Part model, mm, in its own coordinate system. A direction names the side the tool comes from. Round coordinates to 2 decimals unless told otherwise and drop trailing zeros. Write each loop counter-clockwise with the first axis right and the second up, starting at its lowest first coordinate (ties: lowest second). Pieces come first, ordered by that corner, then holes. Notation, with made-up numbers: M 35,-34.5 L 70,-34.5 A16 ccw 70,-4.5 Z; hole C -36,58.5 d11. An arc over 180 degrees is marked long. Answer as a JSON object with one key per item and string values. Group by question number.
1. Band-saw the part on C-C, the plane x = 15. Write the cut outline in (y, z) (3 decimals), plus the area to 3 significant figures.
2. Drop a flat-ended pin along its axis: pin 1 (6 mm diameter, centred on x = 0, y = 15.875, fed in from -Z). Give the stop position or say it passes through.
3. Which spindle directions (+Z, -Z, +X, -X, +Y, -Y) get a long thin tool onto all of the face, cutting with end or side? Do faces 1 (the face through (49.91, -3.63, 2.18)), 2 (the face through (-6, -17.78, 0)), 3 (the face through (0, -9.525, 4)). Say none if no direction does.
4. Band-saw the part on B-B, the plane x = 26.67. Write the cut outline in (y, z) (3 decimals).
5. Two-plate mould, pull along Z, no slides. Class faces 4 (the face through (43, 1, 3.429)), 5 (the face through (26.015, -15.274, 3.658)), 6 (the face through (6, -17.78, 0)): +Z half, -Z half, draft (parallel to the pull), parting line (faces both ways), or undercut.
6. Drill centre lines: line 1 (Y direction, x = -22.86, z = 3.15) (3 decimals); line 2 (Y direction, x = -17.78, z = 5.25) (3 decimals); line 3 (Y direction, x = 26.67, z = 3.8) (3 decimals). Where is each one in solid material? Low to high. Write a range as from..to.
7. Band-saw the part on A-A, the plane x = 0. Write the cut outline in (y, z) (3 decimals), plus the area to 3 significant figures.
8. Band-saw the part on D-D, the plane y = -2. Write the cut outline in (x, z) (3 decimals).
from build123d import *

# Parameters (mm, degrees)
F1_DEPTH  = 6.35
F2_W      = 50.8
F2_H      = 19.05
F2_R      = 5.08
F2_R_2    = 3.175
F2_R_3    = 0.635
F2_R_4    = 1.905
F2_R_5    = 1.27
F2_R_6    = 0.889
F3_DEPTH  = 12.7
F4_W      = 35.56
F4_H      = 1.778
F5_DEPTH  = 76.2
F6_W      = 10.16
F6_H      = 2.54
F7_DEPTH  = 10.16
F8_R      = 5.07999
F9_R      = 3.175
F10_DEPTH = 25.4


# Not quite as in the source:
# - a fillet or chamfer is up to 0.001 mm smaller than in the source, because OpenCascade refuses the exact size


with BuildPart() as f1:
    # F0 (on Top) → F1 (new body, symmetric)
    with BuildSketch(Plane.XY):
        with BuildLine():
            Line((38.735, 22.225), (-38.735, 22.225))
            ThreePointArc((-38.735, 22.225), (-40.5310512242, 21.4810512242), (-41.275, 19.685))
            Line((-41.275, 19.685), (-41.275, -19.685))
            ThreePointArc((-41.275, -19.685), (-40.5310512242, -21.4810512242), (-38.735, -22.225))
            Line((-38.735, -22.225), (38.735, -22.225))
            ThreePointArc((38.735, -22.225), (40.5310512242, -21.4810512242), (41.275, -19.685))
            Line((41.275, -19.685), (41.275, 19.685))
            ThreePointArc((41.275, 19.685), (40.5310512242, 21.4810512242), (38.735, 22.225))
        make_face()
    extrude(amount=F1_DEPTH, both=True)

    # F2 (on face) → F3 (cut, through all)
    with BuildSketch(Plane.XY.offset(6.35)):
        Rectangle(F2_W, F2_H)
        with Locations((0, 15.875)):
            Circle(F2_R)
        with Locations((-10.16, 15.875)):
            Circle(F2_R_2)
        with Locations((-29.972, 15.875)):
            Circle(F2_R_3)
        with Locations((-17.78, 15.875)):
            Circle(F2_R_4)
        with Locations((-22.86, 15.875)):
            Circle(F2_R_5)
        with Locations((-26.67, 15.875)):
            Circle(F2_R_6)
        with Locations((29.972, 15.875)):
            Circle(F2_R_3)
        with Locations((22.86, 15.875)):
            Circle(F2_R_5)
        with Locations((26.67, 15.875)):
            Circle(F2_R_6)
        with Locations((17.78, 15.875)):
            Circle(F2_R_4)
        with Locations((10.16, 15.875)):
            Circle(F2_R_2)
        with Locations((29.972, -15.875)):
            Circle(F2_R_3)
        with Locations((0, -15.875)):
            Circle(F2_R)
        with Locations((26.67, -15.875)):
            Circle(F2_R_6)
        with Locations((-22.86, -15.875)):
            Circle(F2_R_5)
        with Locations((-29.972, -15.875)):
            Circle(F2_R_3)
        with Locations((22.86, -15.875)):
            Circle(F2_R_5)
        with Locations((17.78, -15.875)):
            Circle(F2_R_4)
        with Locations((-26.67, -15.875)):
            Circle(F2_R_6)
        with Locations((-10.16, -15.875)):
            Circle(F2_R_2)
        with Locations((10.16, -15.875)):
            Circle(F2_R_2)
        with Locations((-17.78, -15.875)):
            Circle(F2_R_4)
    extrude(amount=-F3_DEPTH, mode=Mode.SUBTRACT)

    # F4 (on face) → F5 (cut)
    with BuildSketch(Plane.YZ.offset(41.275)):
        Rectangle(F4_W, F4_H)
    extrude(amount=-F5_DEPTH, mode=Mode.SUBTRACT)

    # F6 (on face) → F7 (join)
    with BuildSketch(Plane.YZ.offset(41.275)):
        with Locations((0, 2.159)):
            Rectangle(F6_W, F6_H)
        with Locations((0, -2.159)):
            Rectangle(F6_W, F6_H)
    extrude(amount=F7_DEPTH)

    # F8 (radius 5.08 in the source; OpenCascade refuses exactly that, so slightly less here)
    f8_edges = [f1.edges().sort_by_distance(p)[0] for p in [
        (51.435, -5.08, 2.159),
        (51.435, 5.08, 2.159),
        (51.435, 5.08, -2.159),
        (51.435, -5.08, -2.159),
        (41.275, -5.08, 2.159),
        (41.275, -5.08, -2.159),
        (41.275, 5.08, 2.159),
        (41.275, 5.08, -2.159),
    ]]
    fillet(f8_edges, radius=F8_R)

    # F9 (on face) → F10 (cut)
    with BuildSketch(Plane.XY.offset(3.429)):
        with Locations((46.355, 0)):
            Circle(F9_R)
    extrude(amount=-F10_DEPTH, mode=Mode.SUBTRACT)


solid = f1.part
Worked answers:
{
 "1": {"outline": "M -22.225,-6.35 L -9.525,-6.35 L -9.525,-0.889 L -17.78,-0.889 L -17.78,0.889 L -9.525,0.889 L -9.525,6.35 L -22.225,6.35 Z; M 9.525,-6.35 L 22.225,-6.35 L 22.225,6.35 L 9.525,6.35 L 9.525,0.889 L 17.78,0.889 L 17.78,-0.889 L 9.525,-0.889 Z", "area": "293 mm^2"},
 "2": {"pin 1": "passes through"},
 "3": {"face 1": "+Z, -Z, +X, -Y", "face 2": "+X", "face 3": "+Z, -Z"},
 "4": {"outline": "M -22.225,-6.35 L -16.764,-6.35 L -16.764,-0.889 L -17.78,-0.889 L -17.78,0.889 L -16.764,0.889 L -16.764,6.35 L -22.225,6.35 Z; M -14.986,-6.35 L 14.986,-6.35 L 14.986,-0.889 L -14.986,-0.889 Z; M -14.986,0.889 L 14.986,0.889 L 14.986,6.35 L -14.986,6.35 Z; M 16.764,-6.35 L 22.225,-6.35 L 22.225,6.35 L 16.764,6.35 L 16.764,0.889 L 17.78,0.889 L 17.78,-0.889 L 16.764,-0.889 Z"},
 "5": {"face 4": "+Z half", "face 5": "draft", "face 6": "undercut"},
 "6": {"line 1": "y = -22.225..-17.145, -14.605..-9.525, 9.525..14.605, 17.145..22.225", "line 2": "y = -22.225..-17.78, -13.97..-9.525, 9.525..13.97, 17.78..22.225", "line 3": "y = -22.225..-16.764, -14.986..14.986, 16.764..22.225"},
 "7": {"outline": "M -22.225,-6.35 L -20.955,-6.35 L -20.955,6.35 L -22.225,6.35 Z; M -10.795,-6.35 L -9.525,-6.35 L -9.525,-0.889 L -10.795,-0.889 Z; M -10.795,0.889 L -9.525,0.889 L -9.525,6.35 L -10.795,6.35 Z; M 9.525,-6.35 L 10.795,-6.35 L 10.795,-0.889 L 9.525,-0.889 Z; M 9.525,0.889 L 10.795,0.889 L 10.795,6.35 L 9.525,6.35 Z; M 20.955,-6.35 L 22.225,-6.35 L 22.225,6.35 L 20.955,6.35 Z", "area": "60.0 mm^2"},
 "8": {"outline": "M -41.275,-6.35 L -25.4,-6.35 L -25.4,-0.889 L -34.925,-0.889 L -34.925,0.889 L -25.4,0.889 L -25.4,6.35 L -41.275,6.35 Z; M 25.4,-6.35 L 41.275,-6.35 L 41.275,-3.429 L 43.889,-3.429 L 43.889,-0.889 L 25.4,-0.889 Z; M 25.4,0.889 L 43.889,0.889 L 43.889,3.429 L 41.275,3.429 L 41.275,6.35 L 25.4,6.35 Z; M 48.821,-3.429 L 51.025,-3.429 L 51.025,-0.889 L 48.821,-0.889 Z; M 48.821,0.889 L 51.025,0.889 L 51.025,3.429 L 48.821,3.429 Z"}
}
